The listing builds one solid part. Answer for the finished solid, in the listing's coordinates (mm). A direction names the side the tool comes from. Coordinates: 2 decimals unless noted, no trailing zeros. Order: outer loops, then holes, each group sorted by start corner. A loop starts at its lowest first (then second) coordinate and runs counter-clockwise, first axis right, second up. Notation, with made-up numbers: M 86.25,56 L 142.25,56 A25 cw 142.25,74 Z; hole C 58,21.25 d11. An arc over 180 degrees is marked long. One line per item, written item: value. Start each with the question number.
Q1. The part is cut by section D-D on z = 0.9. Give the number of separate pieces and of enclosed holes in the cut face, then the cut area to 3 significant figures.
Q2. For faces 4 (the flat face through (25, -27, 6)), 5 (the flat face through (-25, 0, 1)), 6 (the cylindrical face through (-17.5, -17.55, 0.99)), 7 (the flat face through (0, -22, 2)), determine the directions among +Z, -Z, +X, -X, +Y, -Y from which every point of the face is accessible in a straight line to the end or side of a thin tool.
Q3. Straight lines are drawn through the part: line 1 along Y through (x, z) = (25, 2.05); line 2 along Y through (x, z) = (8, 1.4). For each, find the intervals that lie inside material, in ascending order. Write a range as [from, to].
Q4. The part is cut by section B-B on y = 14. Give the vertices of the cut face in (x, z), then the cut area to 3 significant figures.
Q5. Each of these flat-tipped pins is pushed along its axis until it touches: pin 1 Ø2.5 at (x, y) = (25, 25) entering from -Z; pin 2 Ø1 at (x, z) = (3.5, 1) entering from +Y; pin 3 Ø0.6 at (y, z) = (8.5, 0.5) entering from -X; pin 4 Ø0.6 at (y, z) = (-1.5, 0.5) entering from +X. Where does it stop, or does it pass through?
Q6. The part is cut by section A-A on z = 4.05. Give the vertices of the cut face in (x, y), then the cut area to 3 significant figures.
Q7. Determine the mould class of faces 1 (the flat face through (25, 23, 6)), 2 (the flat face through (0, 20, 1)), 3 (the flat face through (25, 0, 1)) for opening direction X: pulls with the +X half, pulls with the -X half, needs draft (parallel to the pull), parting line crosses it, or undercut.
```python
from build123d import *

# Parameters (mm, degrees)
SKETCH1_R           = 1.65
BOSS_EXTRUDE1_DEPTH = 2
SKETCH2_R           = 3.5
SKETCH2_R_2         = 1.65
SKETCH2_R_3         = 1.570665428
BOSS_EXTRUDE2_DEPTH = 4
EXTRUDE_THIN1_START = -6
SKETCH3_R           = 1.75
SKETCH3_R_2         = 1.35
EXTRUDE_THIN1_DEPTH = 6


with BuildPart() as part:
    # Sketch1 → Boss-Extrude1 (new body)
    with BuildSketch(Plane.XY):
        with BuildLine():
            Line((-21.5, 25), (21.5, 25))
            ThreePointArc((21.5, 25), (27.474873734, 27.474873734), (25, 21.5))
            Line((25, 21.5), (25, -21.5))
            ThreePointArc((25, -21.5), (27.474873734, -27.474873734), (21.5, -25))
            Line((21.5, -25), (-21.5, -25))
            ThreePointArc((-21.5, -25), (-27.474873734, -27.474873734), (-25, -21.5))
            Line((-25, -21.5), (-25, 21.5))
            ThreePointArc((-25, 21.5), (-27.474873734, 27.474873734), (-21.5, 25))
        make_face()
        with Locations((-20, 20)):
            Circle(SKETCH1_R, mode=Mode.SUBTRACT)
        with Locations((-25, 25)):
            Circle(SKETCH1_R, mode=Mode.SUBTRACT)
        with Locations((20, 20)):
            Circle(SKETCH1_R, mode=Mode.SUBTRACT)
        with Locations((25, 25)):
            Circle(SKETCH1_R, mode=Mode.SUBTRACT)
        with Locations((25, -25)):
            Circle(SKETCH1_R, mode=Mode.SUBTRACT)
        with Locations((20, -20)):
            Circle(SKETCH1_R, mode=Mode.SUBTRACT)
        with Locations((-20, -20)):
            Circle(SKETCH1_R, mode=Mode.SUBTRACT)
        with Locations((-25, -25)):
            Circle(SKETCH1_R, mode=Mode.SUBTRACT)
        with BuildLine():
            Line((-16.5, 20), (16.5, 20))
            ThreePointArc((16.5, 20), (17.525126266, 17.525126266), (20, 16.5))
            Line((20, 16.5), (20, -16.5))
            ThreePointArc((20, -16.5), (17.525126266, -17.525126266), (16.5, -20))
            Line((16.5, -20), (-16.5, -20))
            ThreePointArc((-16.5, -20), (-17.525126266, -17.525126266), (-20, -16.5))
            Line((-20, -16.5), (-20, 16.5))
            ThreePointArc((-20, 16.5), (-17.525126266, 17.525126266), (-16.5, 20))
        make_face(mode=Mode.SUBTRACT)
    extrude(amount=BOSS_EXTRUDE1_DEPTH)

    # Sketch2 → Boss-Extrude2 (add)
    with BuildSketch(Plane.XY.offset(2)):
        with Locations((-25, 25)):
            Circle(SKETCH2_R)
        with Locations((-25, 25)):
            Circle(SKETCH2_R_2, mode=Mode.SUBTRACT)
        with Locations((25, 25)):
            Circle(SKETCH2_R)
        with Locations((25, 25)):
            Circle(SKETCH2_R_3, mode=Mode.SUBTRACT)
        with Locations((-25, -25)):
            Circle(SKETCH2_R)
        with Locations((-25, -25)):
            Circle(SKETCH2_R_2, mode=Mode.SUBTRACT)
        with Locations((25, -25)):
            Circle(SKETCH2_R)
        with Locations((25, -25)):
            Circle(SKETCH2_R_2, mode=Mode.SUBTRACT)
    extrude(amount=BOSS_EXTRUDE2_DEPTH)

    # Sketch3 → Extrude-Thin1 (add)
    with BuildSketch(Plane.XY.offset(6).offset(EXTRUDE_THIN1_START)):
        with Locations((-25, 25)):
            Circle(SKETCH3_R)
        with Locations((-25, 25)):
            Circle(SKETCH3_R_2, mode=Mode.SUBTRACT)
        with Locations((25, 25)):
            Circle(SKETCH3_R)
        with Locations((25, 25)):
            Circle(SKETCH3_R_2, mode=Mode.SUBTRACT)
        with Locations((25, -25)):
            Circle(SKETCH3_R)
        with Locations((25, -25)):
            Circle(SKETCH3_R_2, mode=Mode.SUBTRACT)
        with Locations((-25, -25)):
            Circle(SKETCH3_R)
        with Locations((-25, -25)):
            Circle(SKETCH3_R_2, mode=Mode.SUBTRACT)
    extrude(amount=EXTRUDE_THIN1_DEPTH)


solid = part.part
```
Output:
1. separate pieces: 1
1. enclosed holes: 9
1. area: 997 mm^2
2. face 4: +Z, +X, -X, +Y, -Y
2. face 5: +Z, -Z, -X
2. face 6: +Z, -Z
2. face 7: +Z
3. line 1: y = [-28.5, -26.35], [-23.65, -21.5], [21.5, 23.65], [26.35, 28.5]
3. line 2: y = [-25, -20], [20, 25]
4. outline: M -25,0 L -20,0 L -20,2 L -25,2 Z; M 20,0 L 25,0 L 25,2 L 20,2 Z
4. area: 20.0 mm^2
5. pin 1: passes through
5. pin 2: stops at y = 25
5. pin 3: stops at x = -25
5. pin 4: stops at x = 25
6. outline: C -25,-25 d7; C -25,25 d7; C 25,-25 d7; C 25,25 d7; hole C -25,-25 d2.7; hole C -25,25 d2.7; hole C 25,-25 d2.7; hole C 25,25 d2.7
6. area: 131 mm^2
7. face 1: needs draft
7. face 2: undercut
7. face 3: pulls with the +X half
